```python
from build123d import *

# Parameters (mm, degrees)
SKETCH1_R                   = 7.4
BOSS_EXTRUDE1_DEPTH         = 5.98
CUT_EXTRUDE1_REACH          = 30.218
SKETCH2_R                   = 2.1
CIRPATTERN1_COUNT           = 4
FILLET1_R                   = 7
CUT_EXTRUDE2_DEPTH          = 11
FILLET2_R                   = 2
CIRPATTERN2_COUNT           = 4
CUT_EXTRUDE3_REACH          = 30.218
SKETCH4_R                   = 2.7
CIRPATTERN3_COUNT           = 2
CIRPATTERN3_ANGLE           = 90
CIRPATTERN3_COPY_1_REACH    = 30.218
CIRPATTERN3_COPY_1_SKETCH_R = 2.7


with BuildPart() as part:
    # Sketch1 → Boss-Extrude1 (new body)
    with BuildSketch(Plane.XY):
        Polygon((-10.5, -10.5), (-10.5, -19.5), (10.5, -19.5), (10.5, 10.5), (-19.5, 10.5), (-19.5, -10.5), align=None)
        Circle(SKETCH1_R, mode=Mode.SUBTRACT)
    extrude(amount=-BOSS_EXTRUDE1_DEPTH)

    # Sketch2 → Cut-Extrude1 (cut, up to next)
    with BuildSketch(Plane(origin=(0, 0, -5.98), x_dir=(-1, 0, 0), z_dir=(0, 0, -1)), mode=Mode.PRIVATE) as cut_extrude1_sk1:
        with Locations((-7.25, 7.25)):
            Circle(SKETCH2_R)
    cut_extrude1_tool1 = extrude(cut_extrude1_sk1.sketch, amount=-CUT_EXTRUDE1_REACH, mode=Mode.PRIVATE) & part.part
    cut_extrude1 = cut_extrude1_tool1.solids().sort_by_distance((7.25, 7.25, -5.98))[0]
    add(cut_extrude1, mode=Mode.SUBTRACT)

    # CirPattern1: Cut-Extrude1 ×4 about axis
    cirpattern1_axis = Axis((0, 0, 0), (0, 0, 1))
    for i in range(1, CIRPATTERN1_COUNT):
        add(cut_extrude1.rotate(cirpattern1_axis, i * 360 / CIRPATTERN1_COUNT), mode=Mode.SUBTRACT)

    # Fillet1
    fillet1_edges = [part.edges().sort_by_distance(p)[0] for p in [
        (-10.5, -10.5, -2.99),
    ]]
    fillet(fillet1_edges, radius=FILLET1_R)

    # Sketch3 → Cut-Extrude2 (cut)
    with BuildSketch(Plane(origin=(0, 0, -5.98), x_dir=(-1, 0, 0), z_dir=(0, 0, -1))):
        with BuildLine():
            ThreePointArc((19.5, -9.125478743), (14.512977444, -7.616043809), (9.767409819, -9.767409819))
            Line((9.767409819, -9.767409819), (12.550252532, -12.550252532))
            ThreePointArc((12.550252532, -12.550252532), (14.821215973, -11.032843272), (17.5, -10.5))
            Line((17.5, -10.5), (19.5, -10.5))
            Line((19.5, -10.5), (19.5, -9.125478743))
        make_face()
        with BuildLine():
            ThreePointArc((17.5, -10.5), (14.821215973, -11.032843272), (12.550252532, -12.550252532))
            Line((12.550252532, -12.550252532), (20.232590181, -20.232590181))
            ThreePointArc((20.232590181, -20.232590181), (21.836708541, -17.8318574), (22.4, -15))
            ThreePointArc((22.4, -15), (21.63551053, -11.724332129), (19.5, -9.125478743))
            Line((19.5, -9.125478743), (19.5, -10.5))
            Line((19.5, -10.5), (17.5, -10.5))
        make_face()
        with BuildLine():
            Line((12.550252532, -12.550252532), (9.767409819, -9.767409819))
            ThreePointArc((9.767409819, -9.767409819), (7.616043809, -14.512977444), (9.125478743, -19.5))
            Line((9.125478743, -19.5), (10.5, -19.5))
            Line((10.5, -19.5), (10.5, -17.5))
            ThreePointArc((10.5, -17.5), (11.032843272, -14.821215973), (12.550252532, -12.550252532))
        make_face()
        with BuildLine():
            Line((20.232590181, -20.232590181), (12.550252532, -12.550252532))
            ThreePointArc((12.550252532, -12.550252532), (11.032843272, -14.821215973), (10.5, -17.5))
            Line((10.5, -17.5), (10.5, -19.5))
            Line((10.5, -19.5), (9.125478743, -19.5))
            ThreePointArc((9.125478743, -19.5), (14.512977444, -22.383956191), (20.232590181, -20.232590181))
        make_face()
    cut_extrude2 = extrude(amount=-CUT_EXTRUDE2_DEPTH, mode=Mode.SUBTRACT)

    # Fillet2
    fillet2_edges = [part.edges().sort_by_distance(p)[0] for p in [
        (10.5, 10.5, -2.99),
    ]]
    fillet(fillet2_edges, radius=FILLET2_R)

    # CirPattern2: Cut-Extrude2 ×4 about axis
    cirpattern2_axis = Axis((0, 0, 0), (0, 0, 1))
    for i in range(1, CIRPATTERN2_COUNT):
        add(cut_extrude2.rotate(cirpattern2_axis, i * 360 / CIRPATTERN2_COUNT), mode=Mode.SUBTRACT)

    # Sketch4 → Cut-Extrude3 (cut, up to next)
    with BuildSketch(Plane.XY, mode=Mode.PRIVATE) as cut_extrude3_sk1:
        with Locations((4, -15)):
            Circle(SKETCH4_R)
    cut_extrude3_tool1 = extrude(cut_extrude3_sk1.sketch, amount=-CUT_EXTRUDE3_REACH, mode=Mode.PRIVATE) & part.part
    cut_extrude3 = cut_extrude3_tool1.solids().sort_by_distance((4, -15, 0))[0]
    add(cut_extrude3, mode=Mode.SUBTRACT)

    # Mirror1: Cut-Extrude3 across plane
    add(cut_extrude3.mirror(Plane(origin=(0, 0, 0), x_dir=(0, 0, 1), z_dir=(1, 0, 0))), mode=Mode.SUBTRACT)

    # CirPattern3: Cut-Extrude3 ×2 about axis
    cirpattern3_axis = Axis((0, 0, -48.426406871), (0, 0, -1))
    for i in range(1, CIRPATTERN3_COUNT):
        add(cut_extrude3.rotate(cirpattern3_axis, i * CIRPATTERN3_ANGLE / (CIRPATTERN3_COUNT - 1)), mode=Mode.SUBTRACT)

    # CirPattern3 copy 1 sketch → CirPattern3 copy 1 (cut, up to next)
    with BuildSketch(Plane(origin=(0, 0, 0), x_dir=(0, 1, 0), z_dir=(0, 0, 1)), mode=Mode.PRIVATE) as cirpattern3_copy_1_sk1:
        with Locations((4, 15)):
            Circle(CIRPATTERN3_COPY_1_SKETCH_R)
    cirpattern3_copy_1_tool1 = extrude(cirpattern3_copy_1_sk1.sketch, amount=-CIRPATTERN3_COPY_1_REACH, mode=Mode.PRIVATE) & part.part
    add(cirpattern3_copy_1_tool1.solids().sort_by_distance((-15, 4, 0))[0], mode=Mode.SUBTRACT)


solid = part.part
```
Source: CAD feature listing. Evaluate the final solid. Frame: model axes, mm. Coordinates: 2 decimals unless noted, no trailing zeros. Order: outer loops, then holes, each group sorted by start corner. A loop starts at its lowest first (then second) coordinate and runs counter-clockwise, first axis right, second up. Notation, with made-up numbers: M 45.5,76.5 L 86.5,76.5 A26 cw 86.5,100.5 Z; hole C 77,-18 d3. An arc over 180 degrees is marked long. Write each question's results on one line, items separated by ' | '. Start each with the question number.
1) Draft query along X for faces 1 (the face through (10.5, 0, -3)), 2 (the face through (0, 10.5, -3)), 3 (the face through (-1.604, -7.224, -2.948)). Return one class per face: released by +X, released by -X, zero draft, split by the parting line, or undercut.
2) Section query C-C (y = -6). Return the cut outline in (x, z), plus the area to 3 significant figures.
3) Line query: line 1 (X direction, y = -3.5, z = -2.7); line 2 (Y direction, x = -2, z = -2.4); line 3 (X direction, y = -8.5, z = -2.5). Output: solid intervals per line, ascending. Write a range as from..to.
4) Section query A-A (y = -15). Return the cut outline in (x, z).
5) Section query D-D (z = -2.4). Give the number of separate pieces and of enclosed holes in the cut face, plus the area to 3 significant figures.
Answers:
1) face 1: released by +X | face 2: zero draft | face 3: undercut
2) outline: M -19.5,-5.98 L -16.81,-5.98 L -16.81,0 L -19.5,0 Z; M -13.19,-5.98 L -8.94,-5.98 L -8.94,0 L -13.19,0 Z; M -5.56,-5.98 L -4.33,-5.98 L -4.33,0 L -5.56,0 Z; M 4.33,-5.98 L 5.56,-5.98 L 5.56,0 L 4.33,0 Z; M 8.94,-5.98 L 10.5,-5.98 L 10.5,0 L 8.94,0 Z | area: 65.5 mm^2
3) line 1: x = -19.5..-17.65, -12.35..-6.52, 6.52..10.5 | line 2: y = -19.5..-16.81, -13.19..-7.12, 7.12..10.5 | line 3: x = -19.5..-18.54, -11.46..-8.94, -5.56..5.56, 8.94..10.5
4) outline: M -7.6,-5.98 L -6.7,-5.98 L -6.7,0 L -7.6,0 Z; M -1.3,-5.98 L 1.3,-5.98 L 1.3,0 L -1.3,0 Z; M 6.7,-5.98 L 7.6,-5.98 L 7.6,0 L 6.7,0 Z
5) separate pieces: 1 | enclosed holes: 9 | area: 409 mm^2
